from build123d import *

# Parameters (mm, degrees)
SKETCH1_R           = 4.7
BOSS_EXTRUDE1_DEPTH = 7
SKETCH2_R           = 3.506998357
CUT_EXTRUDE1_DEPTH  = 7
SKETCH3_R           = 7.330684461
BOSS_EXTRUDE2_DEPTH = 2
CHAMFER1_SIZE       = 1


with BuildPart() as part:
    # Sketch1 → Boss-Extrude1 (new body)
    with BuildSketch(Plane(origin=(0, 0, 0), x_dir=(1, 0, 0), z_dir=(0, 1, 0))):
        Circle(SKETCH1_R)
    extrude(amount=BOSS_EXTRUDE1_DEPTH)

    # Sketch2 → Cut-Extrude1 (cut)
    with BuildSketch(Plane(origin=(0, 7, 0), x_dir=(-1, 0, 0), z_dir=(0, 1, 0))):
        Circle(SKETCH2_R)
    extrude(amount=-CUT_EXTRUDE1_DEPTH, mode=Mode.SUBTRACT)

    # Sketch3 → Boss-Extrude2 (add)
    with BuildSketch(Plane(origin=(0, 7, 0), x_dir=(1, 0, 0), z_dir=(0, 1, 0))):
        Circle(SKETCH3_R)
    extrude(amount=BOSS_EXTRUDE2_DEPTH)

    # Chamfer1
    chamfer1_edges = [part.edges().sort_by_distance(p)[0] for p in [
        (-7.330684461, 9, 0),
    ]]
    chamfer(chamfer1_edges, length=CHAMFER1_SIZE)


solid = part.part
Design review of the part built by this model. Coordinates are the model's own, in mm. A direction names the side the tool comes from. Give positions to 0.01 mm unless a question says otherwise; leave off trailing zeros. Loops run counter-clockwise (first coordinate to the right, second up) from the corner with the lowest first, then second, coordinate; pieces in that order, holes last. Notation, with made-up numbers: M -2,87 L 11,87 A20 ccw 11,124 Z; hole C 34.25,33.5 d7. An arc over 180 degrees is marked long. One line per question, with ' | ' between items. Start each with the question number.
1. Add section C-C (y = 4.5). Write out the cut boundary in (x, z).
2. The part is to be moulded in two halves that separate along Z. For faces 3 (the face through (-5.82, 7.49, 4.46)), 4 (the face through (0, 9, 0)), 5 (the face through (0, 7, 0)), 6 (the face through (3.5, 3.5, 0.2)), say which applies: released by +Z, released by -Z, zero draft, split by the parting line, or undercut.
3. Insertion check: P1, Ø3.5, axis at x = 1.5, z = -0.5, coming from the -Y side; P2, Ø3, axis at x = -1.5, y = 1, coming from the +Z side; P3, Ø1, axis at y = 2, z = 2, coming from the -X side. Each pin has a flat end and moves straight along its axis. Give the tip position at first contact, or say it passes through.
4. Add section D-D (y = 8.25). Write out the cut boundary in (x, z).
5. Add section B-B (x = 0). Write out the cut boundary in (y, z), plus the area to 3 significant figures.
6. Add section A-A (z = 0). Write out the cut boundary in (x, y).
7. To check wall thickness, follow L1, parallel to Z at x = 0, y = 4.25; L2, parallel to Y at x = 0, z = -4.75; L3, parallel to Z at x = 2, y = 3.75. State the ranges of each line that lie inside material, in increasing order.
8. For faces 1 (the face through (-1.02, 3.45, 4.59)), 2 (the face through (-4, 0, 0)), list the 3-axis set-ups (+Z, -Z, +X, -X, +Y, -Y) from which the entire face can be reached by the end or side of a thin tool; tool diameter is ignored.
Worked out:
1) outline: C 0,0 d9.4; hole C 0,0 d7.01
2) face 3: split by the parting line | face 4: zero draft | face 5: undercut | face 6: undercut
3) P1: stops at y = 7 | P2: stops at z = 4.7 | P3: stops at x = -4.45
4) outline: C 0,0 d14.16
5) outline: M 0,-4.7 L 7,-4.7 L 7,-7.33 L 8,-7.33 L 9,-6.33 L 9,6.33 L 8,7.33 L 7,7.33 L 7,4.7 L 0,4.7 L 0,3.51 L 7,3.51 L 7,-3.51 L 0,-3.51 Z | area: 45.0 mm²
6) outline: M -7.33,7 L -4.7,7 L -4.7,0 L -3.51,0 L -3.51,7 L 3.51,7 L 3.51,0 L 4.7,0 L 4.7,7 L 7.33,7 L 7.33,8 L 6.33,9 L -6.33,9 L -7.33,8 Z
7) L1: z = -4.7 to -3.51, 3.51 to 4.7 | L2: y = 7 to 9 | L3: z = -4.25 to -2.88, 2.88 to 4.25
8) face 1: -Y | face 2: +Z, -Z, +X, -X, -Y
